Here's how the part is built. I have some questions about the finished solid (model axes, mm). Face numbers are marked on the shaded views. Round coordinates to 2 decimals unless told otherwise and drop trailing zeros. Order: outer loops, then holes, each group sorted by start corner. A loop starts at its lowest first (then second) coordinate and runs counter-clockwise, first axis right, second up. Notation, with made-up numbers: M 85.5,48.5 L 126.5,48.5 A14 cw 126.5,67.5 Z; hole C 80,17.25 d5. An arc over 180 degrees is marked long. Write item = value, one per line. Start each with the question number.
Item 1: I want a section at A-A, the plane y = 37.5. List the corners of the cut face in (x, z) for me.
Item 2: Please list where these lines run through material, in increasing order: L1, parallel to Y at x = 290, z = 7.25; L2, parallel to Y at x = 171.5, z = 7.5; L3, parallel to Y at x = 427.5, z = 4.75.
Item 3: I'm going to push flat-ended pins straight in: P1, Ø17.5, axis at x = 290, y = 37.5, coming from the +Z side; P2, Ø1, axis at y = 172, z = 8, coming from the +X side; P3, Ø1, axis at x = 295, z = 10.5, coming from the -Y side. Where does each tip first touch, or does it pass through?
Item 4: We'd pull the mould along Z, two halves only. Please class the marked faces 1 and 2: pulls with the +Z half, pulls with the -Z half, needs draft (parallel to the pull), parting line crosses it, or undercut.
Item 5: I want a section at C-C, the plane z = 2.5. State how many separate pieces and enclosed holes the cut face has, plus the area to 3 significant figures.
Item 6: I want a section at B-B, the plane x = 290. List the corners of the cut face in (y, z) for me.
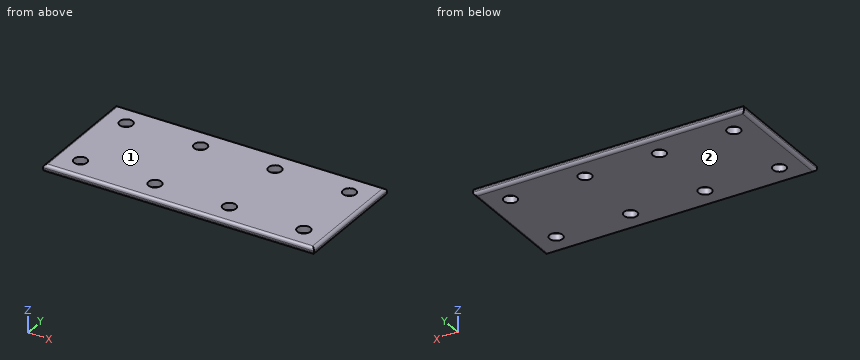
```python
from build123d import *

# Parameters (mm, degrees)
SKETCH_1_W                  = 455
SKETCH_1_H                  = 200
EXTRUDE_1_DEPTH             = 12
SKETCH_2_R                  = 11
CUT_EXTRUDE_2_DEPTH         = 498.160939737
PATTERN_LINEAR_1_COUNT      = 4
PATTERN_LINEAR_1_PITCH      = 125
PATTERN_LINEAR_1_COUNT_DIR2 = 2
PATTERN_LINEAR_1_PITCH_DIR2 = 125
FILLET_1_R                  = 5
FILLET_2_R                  = 5


with BuildPart() as part:
    # 草图1 → 拉伸1 (new body)
    with BuildSketch(Plane.XY):
        with Locations((227.5, 100)):
            Rectangle(SKETCH_1_W, SKETCH_1_H)
    extrude(amount=EXTRUDE_1_DEPTH)

    # 草图2 → 拉伸2 (cut, through all)
    with BuildSketch(Plane.XY.offset(12)):
        with Locations((40, 37.5)):
            Circle(SKETCH_2_R)
    cut_extrude_2 = extrude(amount=-CUT_EXTRUDE_2_DEPTH, mode=Mode.SUBTRACT)

    # 阵列(线性)1: Cut-Extrude 2 4 × 2
    with Locations(*[(i * PATTERN_LINEAR_1_PITCH, j * PATTERN_LINEAR_1_PITCH_DIR2, 0) for i in range(PATTERN_LINEAR_1_COUNT) for j in range(PATTERN_LINEAR_1_COUNT_DIR2) if (i, j) != (0, 0)]):
        add(cut_extrude_2, mode=Mode.SUBTRACT)

    # 圆角1
    fillet_1_edges = [part.edges().sort_by_distance(p)[0] for p in [
        (455, 100, 12),
        (227.5, 200, 12),
        (0, 100, 12),
        (227.5, 0, 12),
    ]]
    fillet(fillet_1_edges, radius=FILLET_1_R)

    # 圆角2
    fillet_2_edges = [part.edges().sort_by_distance(p)[0] for p in [
        (227.5, 200, 0),
        (455, 100, 0),
        (227.5, 0, 0),
        (0, 100, 0),
    ]]
    fillet(fillet_2_edges, radius=FILLET_2_R)


solid = part.part
```
Filled in:
q1.outline = M 0,5 A5 ccw 5,0 L 29,0 L 29,12 L 5,12 A5 ccw 0,7 Z; M 51,0 L 154,0 L 154,12 L 51,12 Z; M 176,0 L 279,0 L 279,12 L 176,12 Z; M 301,0 L 404,0 L 404,12 L 301,12 Z; M 426,0 L 450,0 A5 ccw 455,5 L 455,7 A5 ccw 450,12 L 426,12 Z
q2.L1 = 0.01 to 26.5, 48.5 to 151.5, 173.5 to 199.99
q2.L2 = 0.03 to 28.63, 46.37 to 153.63, 171.37 to 199.97
q2.L3 = 0.01 to 199.99
q3.P1 = through
q3.P2 = 454.97
q3.P3 = 1
q4.face_1 = pulls with the +Z half
q4.face_2 = pulls with the -Z half
q5.separate_pieces = 1
q5.enclosed_holes = 8
q5.area = 87,100 mm^2
q6.outline = M 0,5 A5 ccw 5,0 L 26.5,0 L 26.5,12 L 5,12 A5 ccw 0,7 Z; M 48.5,0 L 151.5,0 L 151.5,12 L 48.5,12 Z; M 173.5,0 L 195,0 A5 ccw 200,5 L 200,7 A5 ccw 195,12 L 173.5,12 Z
